Can you work these out from the drawing? Everything is in mm from the part's minimum corner. A direction names the side the tool comes from. Give positions to 0.01 mm unless a question says otherwise; leave off trailing zeros. Write each loop counter-clockwise with the first axis right and the second up, starting at its lowest first coordinate (ties: lowest second). Pieces come first, ordered by that corner, then holes. Notation, with made-up numbers: (75, -7) - (132, -7) arc R29 ccw to (132, 30) - close; hole circle Ø3 at (-6.5, 21.5). An arc over 180 degrees is marked (long way). Return JSON: item names as keys, results as strings. Group by question number.
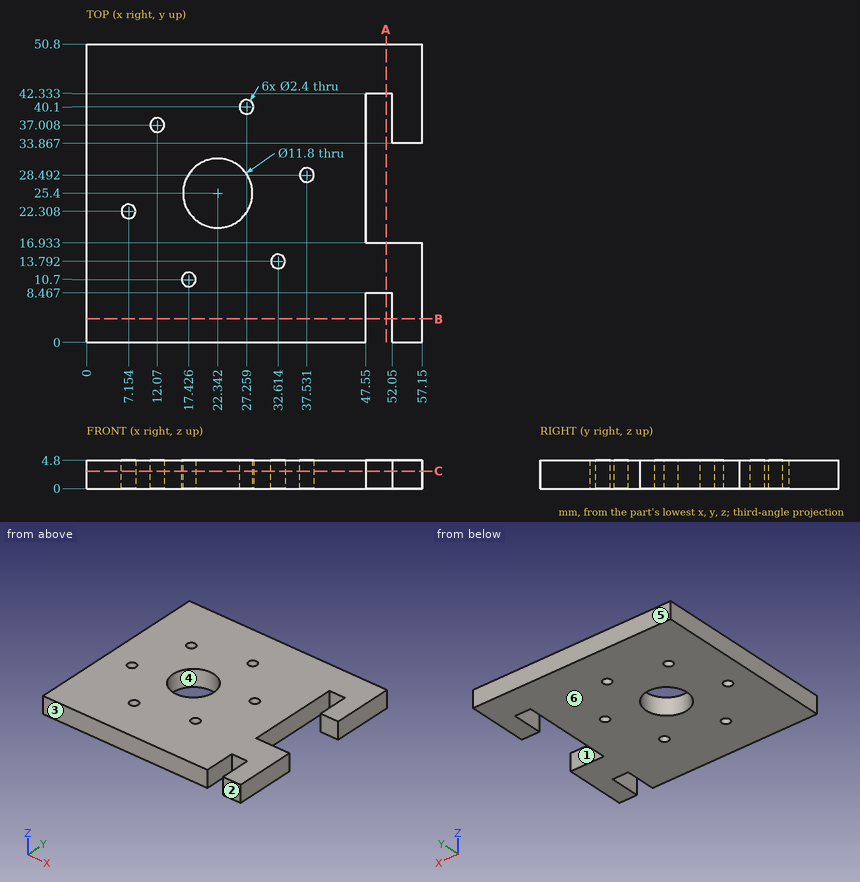
1) Imagine slicing it at C-C, the plane z = 2.95. Count the separate pieces of the cut face and the enclosed holes in it, and give its area (3 significant figures).
2) We'd pull the mould along Y, two halves only. Please class the marked faces 3, 4, 5 and 6: pulls with the +Y half, pulls with the -Y half, needs draft (parallel to the pull), parting line crosses it, or undercut.
3) Will this pin go through, and if not, where does the flat tip stop? pin 1 Ø2.5 at (x, z) = (50.5, 3) entering from -Y.
4) On a 3-axis mill with a long thin cutter (end or side, diameter ignored), from which of +Z, -Z, +X, -X, +Y, -Y can I reach the whole of each face in a straight line? I mean the marked faces 1 and 2. Say none if no direction works.
5) I need wall thicknesses on line 1 along X through (y, z) = (2, 3.35); line 2 along Y through (x, z) = (55, 2.35); line 3 along Y through (x, z) = (52, 4.3). Which ranges of each line are inside material? Lowest first, please.
6) Imagine slicing it at A-A, the plane x = 51. Write out the boundary of the cut face in (y, z).
7) Imagine slicing it at B-B, the plane y = 4. Write out the boundary of the cut face in (x, z).
Resolved:
{
 "1": {"separate pieces": "1", "enclosed holes": "7", "area": "2,530 mm^2"},
 "2": {"face 3": "pulls with the -Y half", "face 4": "undercut", "face 5": "pulls with the +Y half", "face 6": "needs draft"},
 "3": {"pin 1": "y = 8.47"},
 "4": {"face 1": "+Z, -Z, +X", "face 2": "+Z, -Z, +X, -X, -Y"},
 "5": {"line 1": "0 to 47.55, 52.05 to 57.15", "line 2": "0 to 16.93, 33.87 to 50.8", "line 3": "8.47 to 16.93, 42.33 to 50.8"},
 "6": {"outline": "(8.47, 0) - (16.93, 0) - (16.93, 4.8) - (8.47, 4.8) - close; (42.33, 0) - (50.8, 0) - (50.8, 4.8) - (42.33, 4.8) - close"},
 "7": {"outline": "(0, 0) - (47.55, 0) - (47.55, 4.8) - (0, 4.8) - close; (52.05, 0) - (57.15, 0) - (57.15, 4.8) - (52.05, 4.8) - close"}
}
